```python
from build123d import *

# Parameters (mm, degrees)
SKETCH_1_W          = 40
SKETCH_1_H          = 60
EXTRUDE_1_DEPTH     = 5
SKETCH_2_W          = 40
SKETCH_2_H          = 17
EXTRUDE_2_DEPTH     = 12
SKETCH_3_R          = 5.5
CUT_EXTRUDE_1_DEPTH = 15
SKETCH_4_R          = 3
CUT_EXTRUDE_2_DEPTH = 10
SKETCH_7_W          = 20
SKETCH_7_H          = 33
EXTRUDE_4_DEPTH     = 8
SKETCH_8_W          = 10
SKETCH_8_H          = 30
CUT_EXTRUDE_3_DEPTH = 10
SKETCH_9_W          = 10
SKETCH_9_H          = 4
CUT_EXTRUDE_4_DEPTH = 10
SKETCH_10_W         = 10
SKETCH_10_H         = 4
CUT_EXTRUDE_5_DEPTH = 25
CHAMFER_1_SIZE      = 1


with BuildPart() as part:
    # 草图1 → 凸台-拉伸1 (new body)
    with BuildSketch(Plane.XY):
        Rectangle(SKETCH_1_W, SKETCH_1_H)
    extrude(amount=EXTRUDE_1_DEPTH)

    # 草图2 → 凸台-拉伸2 (add)
    with BuildSketch(Plane(origin=(0, 0, 0), x_dir=(-1, 0, 0), z_dir=(0, 0, -1))):
        with Locations((0, -21.5)):
            Rectangle(SKETCH_2_W, SKETCH_2_H)
    extrude(amount=EXTRUDE_2_DEPTH)

    # 草图3 → 切除-拉伸1 (cut)
    with BuildSketch(Plane.XY.offset(5)):
        with Locations((-12, -20)):
            Circle(SKETCH_3_R)
        with Locations((12, -20)):
            Circle(SKETCH_3_R)
    extrude(amount=-CUT_EXTRUDE_1_DEPTH, mode=Mode.SUBTRACT)

    # 草图4 → 切除-拉伸2 (cut)
    with BuildSketch(Plane.XY.offset(-10)):
        with Locations((-12, -20)):
            Circle(SKETCH_4_R)
        with Locations((12, -20)):
            Circle(SKETCH_4_R)
    extrude(amount=-CUT_EXTRUDE_2_DEPTH, mode=Mode.SUBTRACT)

    # 草图7 → 凸台-拉伸4 (add)
    with BuildSketch(Plane.XY.offset(5)):
        with Locations((0, 12.5)):
            Rectangle(SKETCH_7_W, SKETCH_7_H)
    extrude(amount=EXTRUDE_4_DEPTH)

    # 草图8 → 切除-拉伸3 (cut)
    with BuildSketch(Plane(origin=(0, 0, 0), x_dir=(-1, 0, 0), z_dir=(0, 0, -1))):
        with Locations((0, 12)):
            Rectangle(SKETCH_8_W, SKETCH_8_H)
    extrude(amount=-CUT_EXTRUDE_3_DEPTH, mode=Mode.SUBTRACT)

    # 草图9 → 切除-拉伸4 (cut)
    with BuildSketch(Plane.XZ.offset(4)):
        with Locations((0, 7)):
            Rectangle(SKETCH_9_W, SKETCH_9_H)
    extrude(amount=-CUT_EXTRUDE_4_DEPTH, mode=Mode.SUBTRACT)

    # 草图10 → 切除-拉伸5 (cut)
    with BuildSketch(Plane.XY.offset(5)):
        with Locations((-12, -28)):
            Rectangle(SKETCH_10_W, SKETCH_10_H)
    extrude(amount=-CUT_EXTRUDE_5_DEPTH, mode=Mode.SUBTRACT)

    # 倒角1
    chamfer_1_edges = [part.edges().sort_by_distance(p)[0] for p in [
        (-17, -30, -3.5),
        (-17, -26, -3.5),
        (-7, -26, -3.5),
        (-7, -30, -3.5),
    ]]
    chamfer(chamfer_1_edges, length=CHAMFER_1_SIZE)


solid = part.part
```
Geometry check sheet. Reference: the model listing, model coordinates, mm. A direction names the side the tool comes from. Round coordinates to 2 decimals unless told otherwise and drop trailing zeros. Loops run counter-clockwise (first coordinate to the right, second up) from the corner with the lowest first, then second, coordinate; pieces in that order, holes last. Notation, with made-up numbers: (-22.75, 63) -> (16.25, 63) arc R16 ccw to (16.25, 85) -> close; hole circle Ø9 at (39, -25.75). An arc over 180 degrees is marked (long way). Use a Markdown table: item, result.
(1) Sectioned sample at A-A (x = -12). Enter the section's corners in (y, z).
Calculated:
| item | result |
|---|---|
| outline | (-26, -12) -> (-23, -12) -> (-23, -10) -> (-25.5, -10) -> (-25.5, 5) -> (-26, 5) -> close; (-17, -12) -> (-13, -12) -> (-13, 0) -> (30, 0) -> (30, 5) -> (-14.5, 5) -> (-14.5, -10) -> (-17, -10) -> close |
(2) Sectioned sample at B-B (y = -20). Enter the section's corners in (x, z), then the cut area to 3 significant figures.
Calculated:
| item | result |
|---|---|
| outline | (-20, -12) -> (-15, -12) -> (-15, -10) -> (-17.5, -10) -> (-17.5, 5) -> (-20, 5) -> close; (-9, -12) -> (9, -12) -> (9, -10) -> (6.5, -10) -> (6.5, 5) -> (-6.5, 5) -> (-6.5, -10) -> (-9, -10) -> close; (15, -12) -> (20, -12) -> (20, 5) -> (17.5, 5) -> (17.5, -10) -> (15, -10) -> close |
| area | 326 mm² |
(3) Sectioned sample at C-C (z = -4.75). Enter the section's corners in (x, y).
Calculated:
| item | result |
|---|---|
| outline | (-20, -30) -> (-18, -30) -> (-17, -29) -> (-17, -27) -> (-16, -26) -> (-8, -26) -> (-7, -27) -> (-7, -29) -> (-6, -30) -> (20, -30) -> (20, -13) -> (-20, -13) -> close; hole circle Ø11 at (-12, -20); hole circle Ø11 at (12, -20) |
(4) Scan lines: probe 1 along Y at (x, z) = (12, -10.65); probe 2 along Y at (x, z) = (-12, -9.75); probe 3 along Z at (x, y) = (-3.5, -3.5). Record each from-to range of solid material in increasing order.
Calculated:
| item | result |
|---|---|
| probe 1 | -30 to -23, -17 to -13 |
| probe 2 | -26 to -25.5, -14.5 to -13 |
| probe 3 | 0 to 5, 9 to 13 |
(5) Go/stop test with flat-tipped pins: P1, Ø10, axis at x = 12, y = -20, coming from the +Z side; P2, Ø5, axis at x = 12, y = -20, coming from the +Z side; P3, Ø12, axis at x = -7, y = -1, coming from the -Z side; P4, Ø5, axis at y = -3.5, z = 6, coming from the +X side. Record where each tip stops, or that it passes through.
Calculated:
| item | result |
|---|---|
| P1 | z = -10 |
| P2 | through |
| P3 | z = 0 |
| P4 | x = 20 |
(6) Mould release check, pull along X, two halves, no side actions. Record for faces 6 (the flat face through (0, -3, 2)), 7 (the flat face through (-12, -26, -3)), 8 (the flat face through (0, 30, 2)), 9 (the flat face through (10, 12, 9)): released by +X, released by -X, zero draft, split by the parting line, or undercut.
Calculated:
| item | result |
|---|---|
| face 6 | undercut |
| face 7 | undercut |
| face 8 | zero draft |
| face 9 | released by +X |
(7) Sectioned sample at D-D (x = -4). Enter the section's corners in (y, z).
Calculated:
| item | result |
|---|---|
| outline | (-30, -12) -> (-13, -12) -> (-13, 0) -> (-3, 0) -> (-3, 5) -> (-30, 5) -> close; (-4, 9) -> (-3, 9) -> (-3, 10) -> (27, 10) -> (27, 0) -> (30, 0) -> (30, 5) -> (29, 5) -> (29, 13) -> (-4, 13) -> close |
(8) Set-up check for faces 1 (the flat face through (9, 9, 0)), 2 (the flat face through (0, -21, -12)), 3 (the flat face through (20, -7.1, 0.4)), 4 (the cylindrical face through (17.246, -18.348, -2.395)), 5 (the flat face through (-17, -28, -3)): record each of +Z, -Z, +X, -X, +Y, -Y from which the full face is reachable in a straight line by a thin tool's end or side.
Calculated:
| item | result |
|---|---|
| face 1 | -Z, +X, -X, +Y |
| face 2 | -Z, +X, -X, +Y, -Y |
| face 3 | +Z, -Z, +X, +Y, -Y |
| face 4 | +Z |
| face 5 | +Z, -Z, -Y |
